The model under review builds one solid part; all positions refer to its coordinate system, in mm. A direction names the side the tool comes from. Give positions to 0.01 mm unless a question says otherwise; leave off trailing zeros. Order: outer loops, then holes, each group sorted by start corner. A loop starts at its lowest first (then second) coordinate and runs counter-clockwise, first axis right, second up.
Autodesk Inventor part; units mm, degrees
ref_plane "YZ Plane" through (0, 0, 0) normal (1, 0, 0) x (0, 1, 0)
ref_plane "XZ Plane" through (0, 0, 0) normal (0, 1, 0) x (-1, 0, 0)
ref_plane "XY Plane" through (0, 0, 0) normal (0, 0, 1) x (1, 0, 0)
sketch "Sketch1" plane through (0, 0, 0) normal (0, 1, 0) x (-1, 0, 0)
  line L0 (0, 0) -> (-91.4, 0)
  line L1 (-91.4, 0) -> (-91.4, -62.9)
  line L2 (-91.4, -62.9) -> (0, -62.9)
  line L3 (0, -62.9) -> (0, 0)
  line L4 (10, 10) -> (-101.4, 10)
  line L5 (-101.4, 10) -> (-101.4, -72.9)
  line L6 (-101.4, -72.9) -> (10, -72.9)
  line L7 (10, -72.9) -> (10, 10)
  dimension "d0" = 91.4
  dimension "d1" = 62.9
  dimension "d4" = 10
extrude "Extrusion1" add sketch "Sketch1" along normal blind 10
sketch "Sketch2" plane through (0, 0, 0) normal (0, -1, 0) x (1, 0, 0)
  line L0 (101.4, 10) -> (101.4, -72.9)
  line L1 (101.4, -72.9) -> (-10, -72.9)
  line L2 (-10, -72.9) -> (-10, 10)
  line L3 (-10, 10) -> (101.4, 10)
  point P0 (0, 0)
extrude "Extrusion2" add sketch "Sketch2" along normal blind 0.3
fillet "Fillet1" radius 10 4 edges at (-10, 4.85, -72.9) (101.4, 4.85, -72.9) (101.4, 4.85, 10) (-10, 4.85, 10)
sketch "Sketch5" plane through (0, -0.3, 0) normal (0, -1, 0) x (1, 0, 0)
  arc A0 (0, 10) -> (-10, 0) centre (0, 0) ccw
  line L0 (-10, 0) -> (-10, -62.9)
  arc A1 (-10, -62.9) -> (0, -72.9) centre (0, -62.9) ccw
  line L1 (0, -72.9) -> (91.4, -72.9)
  arc A2 (91.4, -72.9) -> (101.4, -62.9) centre (91.4, -62.9) ccw
  line L2 (101.4, -62.9) -> (101.4, 0)
  arc A3 (101.4, 0) -> (91.4, 10) centre (91.4, 0) ccw
  line L3 (91.4, 10) -> (0, 10)
  line L4 (91.4, 0) -> (0, 0)
  line L5 (91.4, -62.9) -> (91.4, 0)
  line L6 (0, -62.9) -> (91.4, -62.9)
  line L7 (0, 0) -> (0, -62.9)
  line L8 (-2.5102, 4.5608) -> (-1.9699, 5.1011)
  circle A4 centre (-3.5355, 3.5355) radius 1.45
  line L9 (45.7, 0) -> (45.7, -31.45)
  line L10 (93.635, 4.1768) -> (91.995, 4.9855)
  circle A5 centre (94.9355, 3.5355) radius 1.45
  line L11 (95.8901, -65.4809) -> (96.3855, -64.9855)
  line L12 (-4.4901, -65.4809) -> (-4.9855, -64.9855)
  circle A6 centre (-3.5355, -66.4355) radius 1.35
  circle A7 centre (94.9355, -66.4355) radius 1.35
  line L13 (0, 0) -> (-2.5102, 2.5102)
  line L14 (-4.5608, 4.5608) -> (-7.0711, 7.0711)
  line L15 (91.4, 0) -> (93.9102, 2.5102)
  line L16 (95.9608, 4.5608) -> (98.4711, 7.0711)
  line L17 (91.4, -62.9) -> (93.9809, -65.4809)
  line L18 (95.8901, -67.3901) -> (98.4711, -69.9711)
  line L19 (0, -62.9) -> (-2.5809, -65.4809)
  line L20 (-4.4901, -67.3901) -> (-7.0711, -69.9711)
extrude "Extrusion3" cut sketch "Sketch5" against normal blind 16 contours A4 | A5 | A6 | A7
sketch "Sketch6" plane through (0, -0.3, 0) normal (0, -1, 0) x (1, 0, 0)
  circle A0 centre (94.9355, -66.4355) radius 1.35
  circle A1 centre (94.9355, 3.5355) radius 1.45
  circle A2 centre (-3.5355, -66.4355) radius 1.35
  circle A3 centre (-3.5355, 3.5355) radius 1.45
  arc A4 (0, 10) -> (-10, 0) centre (0, 0) ccw
  line L0 (-10, 0) -> (-10, -62.9)
  arc A5 (-10, -62.9) -> (0, -72.9) centre (0, -62.9) ccw
  line L1 (0, -72.9) -> (91.4, -72.9)
  arc A6 (91.4, -72.9) -> (101.4, -62.9) centre (91.4, -62.9) ccw
  line L2 (101.4, -62.9) -> (101.4, 0)
  arc A7 (101.4, 0) -> (91.4, 10) centre (91.4, 0) ccw
  line L3 (91.4, 10) -> (0, 10)
  circle A8 centre (-3.5355, -66.4355) radius 2.85
  circle A9 centre (-3.5355, 3.5355) radius 2.95
  circle A10 centre (94.9355, 3.5355) radius 2.95
  circle A11 centre (94.9355, -66.4355) radius 2.85
  point P0 (0, 0)
  dimension "d16" = 1.5
  dimension "d17" = 1.5
  dimension "d18" = 1.5
  dimension "d19" = 1.5
extrude "Extrusion4" add sketch "Sketch6" along normal blind 4 contours L3 A7 L2 A6 L1 A5 L0 A4
sketch "Sketch7" plane through (91.4, 10, -72.9) normal (0, 0, -1) x (-1, 0, 0)
  line L0 (88.212, -2.095) -> (88.212, -9.4812)
  line L1 (88.212, -9.4812) -> (72.9957, -9.4812)
  line L2 (72.9957, -9.4812) -> (72.9957, -2.095)
  line L3 (88.212, -2.095) -> (88.212, -3.345)
  line L4 (72.9957, -3.345) -> (72.9957, -2.095)
  line L5 (88.212, -9.4812) -> (72.9957, -9.4812)
  line L6 (72.9957, -9.4812) -> (72.9957, -1.4812)
  line L7 (72.9957, -1.4812) -> (88.212, -1.4812)
  line L8 (88.212, -1.4812) -> (88.212, -9.4812)
  point P0 (91.4, -10)
  dimension "d24" = 1.25
extrude "Extrusion5" cut sketch "Sketch7" against normal blind 44.15
fillet "Fillet2" radius 3 4 edges at (18.4043, 0.5188, -67.9) (3.188, 0.5188, -67.9) (18.4043, 8.5188, -67.9) (3.188, 8.5188, -67.9)
properties part number "Bottom"
1. Draft analysis for pull direction X (two halves, no side actions). For faces 1 (the flat face through (45, 3, -72.9)), 2 (the cylindrical face through (4.043, 1.421, -67.83)), 3 (the flat face through (101.4, 3, -32)), state which applies: pulls with the +X half, pulls with the -X half, needs draft (parallel to the pull), parting line crosses it, or undercut.
2. Take a section at B-B (y = -1.5). Write out the cut boundary in (x, z).
3. To check wall thickness, follow line 1 (X direction, y = 3.5, z = -53); line 2 (Z direction, x = 23.5, y = 7.5); line 3 (Z direction, x = 96, y = 1.5). State the ranges of each line that lie inside material, in increasing order.
4. Take a section at A-A (z = -22). Write out the cut boundary in (x, y), and give its area (3 significant figures).
5. For faces 4 (the cylindrical face through (4.09, 7.663, -67.83)), 5 (the cylindrical face through (-3.711, 4.778, -65.097)), 6 (the flat face through (96, -0.3, 5)), 7 (the flat face through (0, 5, -32)), list the 3-axis set-ups (+Z, -Z, +X, -X, +Y, -Y) from which the entire face can be reached by the end or side of a thin tool; tool diameter is ignored.
6. Insertion check: pin 1 (5.5 mm diameter, centred on x = 94.94, z = 3.54, fed in from +Y); pin 2 (2 mm diameter, centred on y = 5, z = -70, fed in from +X); pin 3 (4 mm diameter, centred on x = -3.54, z = 3.54, fed in from -Y); pin 4 (1 mm diameter, centred on y = 4, z = -69, fed in from -X). Each pin has a flat end and moves straight along its axis. Give the tip position at first contact, or say it passes through.
7. Take a section at C-C (x = 38). Write out the cut boundary in (y, z).
Answer:
1. face 1: needs draft
1. face 2: undercut
1. face 3: pulls with the +X half
2. outline: (-10, -62.9) arc R10 ccw to (0, -72.9) - (91.4, -72.9) arc R10 ccw to (101.4, -62.9) - (101.4, 0) arc R10 ccw to (91.4, 10) - (0, 10) arc R10 ccw to (-10, 0) - close; hole circle Ø5.9 at (-3.54, 3.54); hole circle Ø5.7 at (-3.54, -66.44); hole circle Ø5.9 at (94.94, 3.54); hole circle Ø5.7 at (94.94, -66.44)
3. line 1: x = -10 to 0, 91.4 to 101.4
3. line 2: z = -72.9 to -62.9, 0 to 10
3. line 3: z = -71.78 to -67.27, -65.61 to 2.55, 4.52 to 8.88
4. outline: (-10, -4.3) - (101.4, -4.3) - (101.4, 10) - (91.4, 10) - (91.4, 0) - (0, 0) - (0, 10) - (-10, 10) - close
4. area: 679 mm2
5. face 4: -Z
5. face 5: +Y, -Y
5. face 6: -Y
5. face 7: +Y
6. pin 1: stops at y = 10
6. pin 2: stops at x = 99.32
6. pin 3: stops at y = -0.3
6. pin 4: stops at x = -8.28
7. outline: (-4.3, -72.9) - (10, -72.9) - (10, -62.9) - (0, -62.9) - (0, 0) - (10, 0) - (10, 10) - (-4.3, 10) - close
